from build123d import *

# Parameters (mm, degrees)
BOSS_EXTRUDE1_DEPTH = 3.2
SKETCH2_W           = 4.8
SKETCH2_H           = 3.3
CUT_EXTRUDE1_DEPTH  = 8.9
SKETCH3_R           = 1.125
CUT_EXTRUDE2_DEPTH  = 2
SKETCH4_R           = 2.4
CUT_EXTRUDE3_DEPTH  = 5


with BuildPart() as part:
    # Sketch1 → Boss-Extrude1 (new, symmetric)
    with BuildSketch(Plane(origin=(0, 0, 0), x_dir=(0, 0, -1), z_dir=(1, 0, 0))):
        with BuildLine():
            Line((0, 0), (-7.8, 0))
            Line((-7.8, 0), (-7.8, 11.2))
            ThreePointArc((-7.8, 11.2), (-2.734752416, 14.330495168), (-2.2, 8.4))
            Line((-2.2, 8.4), (-2.2, 3.2))
            Line((-2.2, 3.2), (0, 3.2))
            Line((0, 3.2), (0, 0))
        make_face()
    extrude(amount=BOSS_EXTRUDE1_DEPTH, both=True)

    # Sketch2 → Cut-Extrude1 (cut)
    with BuildSketch(Plane.XZ):
        with Locations((0, 4.75)):
            Rectangle(SKETCH2_W, SKETCH2_H)
    extrude(amount=-CUT_EXTRUDE1_DEPTH, mode=Mode.SUBTRACT)

    # Sketch3 → Cut-Extrude2 (cut)
    with BuildSketch(Plane.ZY.offset(3.2)):
        with Locations((4.3, 11.2)):
            Circle(SKETCH3_R)
    extrude(amount=-CUT_EXTRUDE2_DEPTH, mode=Mode.SUBTRACT)

    # Sketch4 → Cut-Extrude3 (cut)
    with BuildSketch(Plane.XY.offset(7.8)):
        with Locations((0, 11.7)):
            Circle(SKETCH4_R)
    extrude(amount=-CUT_EXTRUDE3_DEPTH, mode=Mode.SUBTRACT)


solid = part.part
Design review of the part built by this model. Coordinates are the model's own, in mm. A direction names the side the tool comes from. Give positions to 0.01 mm unless a question says otherwise; leave off trailing zeros. Loops run counter-clockwise (first coordinate to the right, second up) from the corner with the lowest first, then second, coordinate; pieces in that order, holes last. Notation, with made-up numbers: (-19.5, 50) - (11.5, 50) arc R32 cw to (11.5, 78) - close; hole circle Ø8 at (69, 56). An arc over 180 degrees is marked (long way). Write item = value, one per line.
1) To check wall thickness, follow line 1 (Z direction, x = -2.6, y = 11.2) (3 decimals); line 2 (X direction, y = 7.25, z = 5.5); line 3 (Z direction, x = 1, y = 7.25). State the ranges of each line that lie inside material, in increasing order.
Result sheet:
line_1 = 0.8 to 3.175, 5.425 to 7.8
line_2 = -3.2 to -2.4, 2.4 to 3.2
line_3 = 2.2 to 3.1, 6.4 to 7.8
2) Draft analysis for pull direction X (two halves, no side actions). For faces 5 (the face through (3.2, 7, 5)), 6 (the face through (0, 6, 2.2)), 7 (the face through (0, 4, 3.1)), state which applies: +X half, -X half, draft (parallel to the pull), parting line (faces both ways), or undercut.
Result sheet:
face_5 = +X half
face_6 = draft
face_7 = undercut
3) Tool access review of faces 1 (the face through (0, 3.2, 1)), 2 (the face through (0, 4, 6.4)), 3 (the face through (-2.65, 10.1, 4.06)), 4 (the face through (1.11, 9.57, 5.34)): name each direction out of +Z, -Z, +X, -X, +Y, -Y from which nothing blocks a thin tool from reaching the whole face with its end or side.
Result sheet:
face_1 = -Z, +X, -X
face_2 = -Y
face_3 = -X
face_4 = +Z
4) Take a section at A-A on y = 7.5. State the section outline as (x, z) points, and give its area (3 significant figures).
Result sheet:
outline = (-3.2, 2.2) - (3.2, 2.2) - (3.2, 7.8) - (-3.2, 7.8) - close; hole (-2.4, 3.1) - (2.4, 3.1) - (2.4, 6.4) - (-2.4, 6.4) - close
area = 20.0 mm2
5) Take a section at B-B on z = 1.25. State the section outline as (x, y) points, and give its area (3 significant figures).
Result sheet:
outline = (-3.2, 0) - (3.2, 0) - (3.2, 3.2) - (-3.2, 3.2) - close; (-3.2, 9.48) - (3.2, 9.48) - (3.2, 12.92) - (-3.2, 12.92) - close
area = 42.5 mm2
6) Take a section at C-C on x = -1.5. State the section outline as (y, z) points, and give its area (3 significant figures).
Result sheet:
outline = (0, 0) - (3.2, 0) - (3.2, 2.2) - (8.4, 2.2) arc R3.5 ccw (long way) to (13.57, 6.87) - (13.57, 2.8) - (9.83, 2.8) - (9.83, 7.8) - (0, 7.8) - (0, 6.4) - (8.9, 6.4) - (8.9, 3.1) - (0, 3.1) - close
area = 44.3 mm2
7) Take a section at D-D on y = 10.5. State the section outline as (x, z) points, and give its area (3 significant figures).
Result sheet:
outline = (-3.2, 0.87) - (3.2, 0.87) - (3.2, 7.8) - (2.08, 7.8) - (2.08, 2.8) - (-2.08, 2.8) - (-2.08, 3.42) - (-3.2, 3.42) - close; (-3.2, 5.18) - (-2.08, 5.18) - (-2.08, 7.8) - (-3.2, 7.8) - close
area = 21.6 mm2
8) Clearance check with flat-ended pins moving along their axes: pin 1 Ø1.6 at (x, z) = (0, 5.5) entering from -Y; pin 2 Ø1.1 at (x, z) = (-1, 1) entering from +Y; pin 3 Ø2.5 at (x, y) = (0, 5) entering from -Z. State where each tip first meets the part, or that it passes through.
Result sheet:
pin_1 = 8.9
pin_2 = 13.37
pin_3 = 2.2
